```python
from build123d import *

# Parameters (mm, degrees)
BOSS_EXTRUDE1_DEPTH            = 12.7
CUT_EXTRUDE1_DEPTH             = 13.7
SKETCH3_W                      = 18.5
SKETCH3_H                      = 12.7
F_3_7_3_7_DIAMETER_HOLE1_D     = 3.7
F_3_7_3_7_DIAMETER_HOLE1_DEPTH = 6.7
F_3_7_3_7_DIAMETER_HOLE2_D     = 3.7
F_3_7_3_7_DIAMETER_HOLE2_DEPTH = 45
F_3_7_3_7_DIAMETER_HOLE3_D     = 3.7
F_3_7_3_7_DIAMETER_HOLE3_DEPTH = 45
FILLET1_R                      = 1.5
FILLET2_R                      = 6.35


with BuildPart() as part:
    # Sketch1 → Boss-Extrude1 (new body)
    with BuildSketch(Plane.XY.offset(6.35)):
        with BuildLine():
            Line((-20.952565475, 8.2), (-36, 8.2))
            Line((-36, 8.2), (-36, -22.5))
            Line((-36, -22.5), (36, -22.5))
            Line((36, -22.5), (36, 0))
            Line((36, 0), (22.5, 0))
            ThreePointArc((22.5, 0), (4.172366044, 22.109757158), (-20.952565475, 8.2))
        make_face()
    extrude(amount=-BOSS_EXTRUDE1_DEPTH)

    # Sketch2 → Cut-Extrude1 (cut, through all)
    with BuildSketch(Plane(origin=(0, 0, -6.35), x_dir=(-1, 0, 0), z_dir=(0, 0, -1))):
        with BuildLine():
            Line((36, 1.5), (18.439088915, 1.5))
            ThreePointArc((18.439088915, 1.5), (18.5, 0), (18.439088915, -1.5))
            Line((18.439088915, -1.5), (36, -1.5))
            Line((36, -1.5), (36, 1.5))
        make_face()
    extrude(amount=-CUT_EXTRUDE1_DEPTH, mode=Mode.SUBTRACT)

    # Sketch3 → Cut-Revolve1 (revolve, cut)
    with BuildSketch(Plane(origin=(0, 0, 0), x_dir=(1, 0, 0), z_dir=(0, 1, 0))):
        with Locations((9.25, 0)):
            Rectangle(SKETCH3_W, SKETCH3_H)
    revolve(axis=Axis((0, 0, -6.35), (0, 0, 1)), mode=Mode.SUBTRACT)

    # Ø3.7 (3.7) Diameter Hole1
    with Locations(Plane(origin=(0, 8.2, 0), x_dir=(1, 0, 0), z_dir=(0, 1, 0))):
        with Locations((-32, 0)):
            Hole(F_3_7_3_7_DIAMETER_HOLE1_D / 2, depth=F_3_7_3_7_DIAMETER_HOLE1_DEPTH)

    # Ø3.7 (3.7) Diameter Hole2
    with Locations(Plane(origin=(0, -22.5, 0), x_dir=(-1, 0, 0), z_dir=(0, -1, 0))):
        with Locations((32, 0)):
            Hole(F_3_7_3_7_DIAMETER_HOLE2_D / 2, depth=F_3_7_3_7_DIAMETER_HOLE2_DEPTH)

    # Ø3.7 (3.7) Diameter Hole3
    with Locations(Plane(origin=(0, -22.5, 0), x_dir=(-1, 0, 0), z_dir=(0, -1, 0))):
        with Locations((-32, 0)):
            Hole(F_3_7_3_7_DIAMETER_HOLE3_D / 2, depth=F_3_7_3_7_DIAMETER_HOLE3_DEPTH)

    # Fillet1
    fillet1_edges = [part.edges().sort_by_distance(p)[0] for p in [
        (36, 0, 0),
        (-36, 8.2, 0),
    ]]
    fillet(fillet1_edges, radius=FILLET1_R)

    # Fillet2
    fillet2_edges = [part.edges().sort_by_distance(p)[0] for p in [
        (22.5, 0, 0),
        (-20.952565475, 8.2, 0),
    ]]
    fillet(fillet2_edges, radius=FILLET2_R)


solid = part.part
```
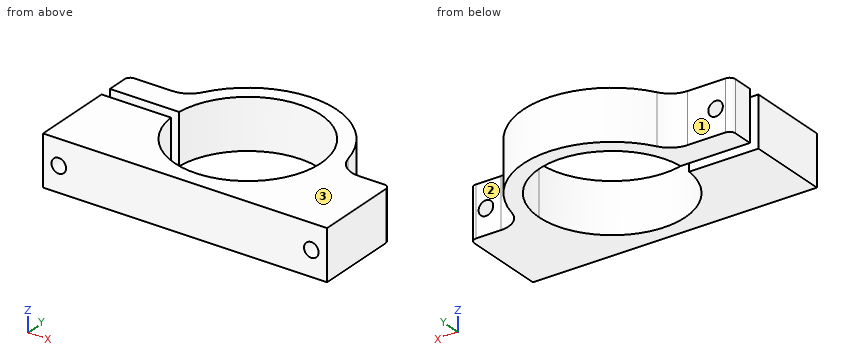
Check sheet for the modelled part. Datum: model origin and axes. Units: mm. Face numbers are marked on the shaded views. A direction names the side the tool comes from. Round coordinates to 2 decimals unless told otherwise and drop trailing zeros. Loops run counter-clockwise (first coordinate to the right, second up) from the corner with the lowest first, then second, coordinate; pieces in that order, holes last. Notation, with made-up numbers: M 43.5,-2 L 83.5,-2 A24 cw 83.5,24 Z; hole C 63,87.25 d11. An arc over 180 degrees is marked long. Answer as a JSON object with one key per item and string values.
1. Section check C-C (y = -12). Record the boundary of the cut face in (x, z), plus the area to 3 significant figures.
Reply:
{"outline": "M -36,-6.35 L -14.08,-6.35 L -14.08,6.35 L -36,6.35 Z; M 14.08,-6.35 L 36,-6.35 L 36,6.35 L 14.08,6.35 Z; hole C -32,0 d3.7; hole C 32,0 d3.7", "area": "535 mm²"}
2. Section check D-D (x = -32). Record the boundary of the cut face in (y, z).
Reply:
{"outline": "M -22.5,-6.35 L -1.5,-6.35 L -1.5,-1.85 L -22.5,-1.85 Z; M -22.5,1.85 L -1.5,1.85 L -1.5,6.35 L -22.5,6.35 Z; M 1.5,-6.35 L 8.2,-6.35 L 8.2,-1.85 L 1.5,-1.85 Z; M 1.5,1.85 L 8.2,1.85 L 8.2,6.35 L 1.5,6.35 Z"}
3. Scan lines: line 1 (Y direction, x = -26, z = 3.5); line 2 (Z direction, x = -32, y = 6.5); line 3 (Y direction, x = 0, z = 2.25). Record each from-to range of solid material in increasing order.
Reply:
{"line 1": "y = -22.5 to -1.5, 1.5 to 8.2", "line 2": "z = -6.35 to -1.85, 1.85 to 6.35", "line 3": "y = -22.5 to -18.5, 18.5 to 22.5"}
4. Section check B-B (x = 0). Record the boundary of the cut face in (y, z), plus the area to 3 significant figures.
Reply:
{"outline": "M -22.5,-6.35 L -18.5,-6.35 L -18.5,6.35 L -22.5,6.35 Z; M 18.5,-6.35 L 22.5,-6.35 L 22.5,6.35 L 18.5,6.35 Z", "area": "102 mm²"}
5. Gauge pin test, flat ends, axial feed: P1, Ø6.5, axis at x = -26.5, z = -2.5, coming from the +Y side; P2, Ø3.5, axis at x = 32, z = 0, coming from the +Y side; P3, Ø3, axis at x = 30.5, z = -2, coming from the +Y side; P4, Ø1, axis at x = 4.5, z = 1, coming from the +Y side. Record the tip position at first contact, or that the pin passes through.
Reply:
{"P1": "stops at y = 8.42", "P2": "passes through", "P3": "stops at y = 0", "P4": "stops at y = 22.14"}
6. Access from +Z, -Z, +X, -X, +Y, -Y to the whole of each face (thin tool, end or side, straight path). Record for the marked faces 1, 2 and 3.
Reply:
{"face 1": "+Z, -Z, -X, +Y", "face 2": "+Z, -Z, +X, +Y", "face 3": "+Z, +X, -X, +Y, -Y"}
7. Section check A-A (z = 0). Record the boundary of the cut face in (x, y), plus the area to 3 significant figures.
Reply:
{"outline": "M -36,-22.5 L -33.85,-22.5 L -33.85,-1.5 L -36,-1.5 Z; M -36,1.5 L -33.85,1.5 L -33.85,8.2 L -34.5,8.2 A1.5 ccw -36,6.7 Z; M -30.15,-22.5 L 30.15,-22.5 L 30.15,0 L 28.14,0 A6.35 cw 21.95,4.95 A22.5 ccw -19.43,11.35 A6.35 cw -24.91,8.2 L -30.15,8.2 L -30.15,1.5 L -18.44,1.5 A18.5 cw long -18.44,-1.5 L -30.15,-1.5 Z; M 33.85,-22.5 L 36,-22.5 L 36,-1.5 A1.5 ccw 34.5,0 L 33.85,0 Z", "area": "1,220 mm²"}
